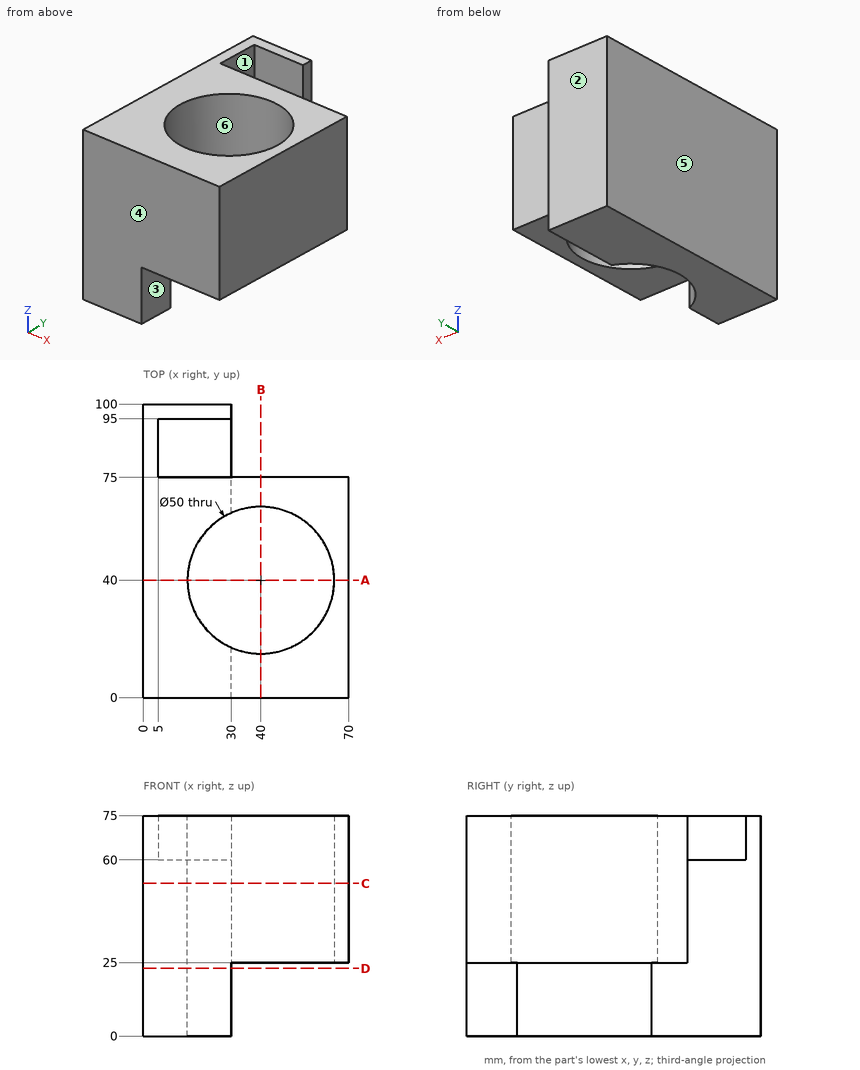
Part print with two shaded views. Sizes in mm from the minimum x, y, z corner. A direction names the side the tool comes from. Round coordinates to 2 decimals unless told otherwise and drop trailing zeros. Loops run counter-clockwise (first coordinate to the right, second up) from the corner with the lowest first, then second, coordinate; pieces in that order, holes last. Notation, with made-up numbers: (-39.5, -6) - (5.5, -6) arc R37 cw to (5.5, 31) - close; hole circle Ø4 at (-38.5, 68). An arc over 180 degrees is marked (long way). Answer as a JSON object with one key per item and string values.
Item 1: Band-saw the part on C-C on z = 52. List the corners of the cut face in (x, y), plus the area to 3 significant figures.
Output:
{"outline": "(0, 0) - (70, 0) - (70, 75) - (30, 75) - (30, 100) - (0, 100) - close; hole circle Ø50 at (40, 40)", "area": "4,040 mm2"}
Item 2: Tool access for the marked faces 1, 2 and 3: list every direction of +Z, -Z, +X, -X, +Y, -Y with a clear straight run to the whole face (end or side of a thin tool).
Output:
{"face 1": "+Z, +X", "face 2": "+Z, -Z, +X, -X, +Y", "face 3": "-Z, +X, +Y, -Y"}
Item 3: Band-saw the part on B-B on x = 40. List the corners of the cut face in (y, z), plus the area to 3 significant figures.
Output:
{"outline": "(0, 25) - (15, 25) - (15, 75) - (0, 75) - close; (65, 25) - (75, 25) - (75, 75) - (65, 75) - close", "area": "1,250 mm2"}
Item 4: Wall check: L1, parallel to X at y = 40, z = 29; L2, parallel to Y at x = 40, z = 48; L3, parallel to Z at x = 39, y = 73. Give the ranges that are in metal, low to high.
Output:
{"L1": "0 to 15, 65 to 70", "L2": "0 to 15, 65 to 75", "L3": "25 to 75"}
Item 5: Band-saw the part on A-A on y = 40. List the corners of the cut face in (x, z), plus the area to 4 significant figures.
Output:
{"outline": "(0, 0) - (15, 0) - (15, 75) - (0, 75) - close; (65, 25) - (70, 25) - (70, 75) - (65, 75) - close", "area": "1,375 mm2"}
Item 6: Pull direction X, two halves, no side cores. Call the marked faces 4, 5 and 6: pulls with the +X half, pulls with the -X half, needs draft (parallel to the pull), parting line crosses it, or undercut.
Output:
{"face 4": "needs draft", "face 5": "pulls with the -X half", "face 6": "undercut"}
Item 7: Pin check, flat tips, straight feed: pin 1 (10 mm diameter, centred on x = 13, y = 87.5, fed in from +Z); pin 2 (11 mm diameter, centred on y = 83, z = 50.5, fed in from +X); pin 3 (4.5 mm diameter, centred on y = 84, z = 66.5, fed in from +X). Stop position of each tip, or through.
Output:
{"pin 1": "z = 60", "pin 2": "x = 30", "pin 3": "x = 5"}
Item 8: Band-saw the part on D-D on z = 23. List the corners of the cut face in (x, y), plus the area to 3 significant figures.
Output:
{"outline": "(0, 0) - (30, 0) - (30, 17.09) arc R25 cw to (30, 62.91) - (30, 100) - (0, 100) - close", "area": "2,500 mm2"}
